Verification items for the finished model (mm, model axes). Face numbers are marked on the shaded views. A direction names the side the tool comes from. Coordinates: 2 decimals unless noted, no trailing zeros. Order: outer loops, then holes, each group sorted by start corner. A loop starts at its lowest first (then second) coordinate and runs counter-clockwise, first axis right, second up. Notation, with made-up numbers: M 10.25,57 L 56.25,57 A25 ccw 56.25,79 Z; hole C 69,65.25 d8. An arc over 180 degrees is marked long. Return JSON: item names as keys, results as strings.
Autodesk Inventor part; units mm, degrees
ref_plane "Work Plane1" through (30, 0, 0) normal (0, -0.5, 0.866) x (1, 0, 0)
ref_plane "YZ Plane" through (0, 0, 0) normal (1, 0, 0) x (0, 1, 0)
ref_plane "XZ Plane" through (0, 0, 0) normal (0, 1, 0) x (-1, 0, 0)
sketch "Skizze1" plane through (0, 0, 0) normal (0, 0, 1) x (1, 0, 0)
  line L0 (-0.19, 0) -> (25, 0)
  line L1 (25, 0) -> (25, 2.5)
  line L2 (25, 2.5) -> (1.6, 2.5)
  line L3 (1.6, 2.5) -> (1.1092, 2.5)
  line L4 (1.1092, 2.5) -> (0, 2.5)
  line L5 (0, 2.5) -> (0, 4.75)
  line L6 (0, 4.75) -> (-2.75, 4.75)
  line L7 (-2.75, 4.75) -> (-2.75, 1.7321)
  line L8 (-2.75, 1.7321) -> (-1.19, 1.7321)
  line L9 (-1.19, 1.7321) -> (-0.19, 0)
  line L10 (-8.3, 0) -> (30.55, 0)
  line L11 (0, -0.95) -> (0, 5.7)
  line L12 (1.6, 2.5) -> (0, 2.5) construction
  dimension "d0" = 23.4
  dimension "d1" = 0.4908
  dimension "d2" = 2.75
  dimension "d3" = 1.56
  dimension "d4" = 60
  dimension "d5" = 5
  dimension "d6" = 5
  dimension "d7" = 3.4641
  dimension "d8" = 9.5
  dimension "d19" = 25
revolve "Körper" add sketch "Skizze1" angle 360 about axis through (-0.19, 0, 0) along (1, 0, 0)
sketch "Skizze2" plane through (-2.75, 0, 0) normal (-1, 0, 0) x (0, 0, 1)
  circle A0 centre (0, 0) radius 1.7321
  line L0 (0, -6.65) -> (0, 6.65)
  line L1 (-6.65, 0) -> (6.65, 0)
  line L2 (1.7321, 0) -> (0.866, -1.5)
  line L3 (0.866, -1.5) -> (-0.866, -1.5)
  line L4 (-0.866, -1.5) -> (-1.7321, 0)
  line L5 (-1.7321, 0) -> (-0.866, 1.5)
  line L6 (-0.866, 1.5) -> (0.866, 1.5)
  line L7 (0.866, 1.5) -> (1.7321, 0)
extrude "Loch" add sketch "Skizze2" against normal up to next contours L7 A0 | A0 L2 | L6 L0 A0 | A0 L0 L3 | L0 L6 A0 | A0 L3 L0 | L4 A0 | A0 L5
fillet "Rundung1" radius 2.375 1 edges at (-2.75, -4.75, 0)
thread "Gewinde"
chamfer "Fase1" distance 0.4908 distance2 0.4908 1 edges at (25, -2.5, 0) measured on face at (25, 0.6587, -0.3326)
fillet "Rundung2" radius 0.2 1 edges at (0, -2.5, 0)
ref_plane "Work Plane1" through (30, 0, 0) normal (0, -0.5, 0.866) x (1, 0, 0)
sketch "Skizze4" plane through (25, 0, 0) normal (1, 0, 0) x (0, 0, -1)
  circle A0 centre (0, 0) radius 5
extrude "Extrusion3" cut sketch "Skizze4" against normal blind 3
chamfer "Fase3" distance 0.5 angle 45 1 edges at (22, -2.5, 0)
equation "\"d0\" = GEL"
equation "\"d1\" = GAL"
equation "\"d2\" = KOH"
equation "\"d3\" = INTI"
equation "\"d5\" = GD"
equation "\"d6\" = BDM"
equation "\"d7\" = 1.1547 * SW"
equation "\"d8\" = KOD"
equation "\"d19\" = NLG"
equation "\"d16\" = RR"
equation "\"d12\" = GEL"
equation "\"d14\" = -0.5 * SPD + 0.5 * GD"
equation "\"d15\" = GUL"
equation "\"d29\" = R"
equation "\"GD\" = NND"
equation "\"NLG\" = 25"
equation "\"GEL\" = 23.4"
equation "\"KOD\" = 9.5"
equation "\"KOH\" = 2.75"
equation "\"INTI\" = 1.56"
equation "\"GAL\" = 0.61345 * PTC"
equation "\"GUL\" = 0.61345 * PTC"
equation "\"BDM\" = NND"
equation "\"SW\" = 3"
equation "\"RR\" = 2.375"
equation "\"SPD\" = 4.01848"
equation "\"d28\" = R"
equation "\"R\" = 0.2"
equation "\"TOA\" = 30deg"
equation "\"THREADDIA\" = 5"
equation "\"KOD1\" = KOD - 2 * RR"
equation "\"PTC\" = 0.8"
equation "\"NND\" = 5"
equation "\"E0\" = 1.155 * SW"
equation "\"GD1\" = THREADDIA - 1.2269 * PTC"
properties part number "ANSI B18.3.4M - M5 x 0.8 x 25, BHSBHCSM" material "Stahl, weich"
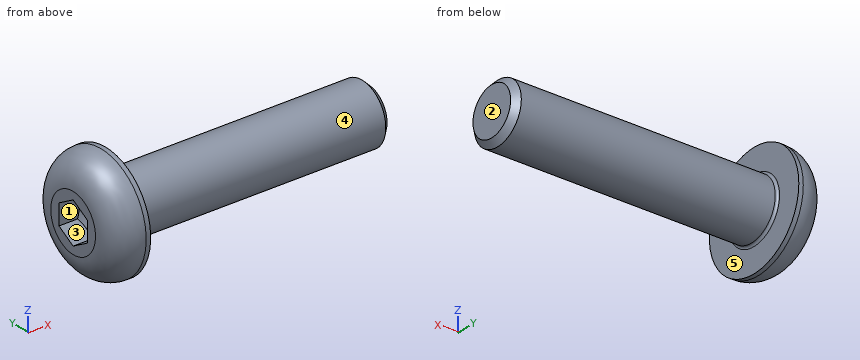
Q1. Draft check along Z on the marked faces 3, 4 and 5. Enter one of: pulls with the +Z half, pulls with the -Z half, needs draft (parallel to the pull), parting line crosses it, or undercut.
Values:
{"face 3": "undercut", "face 4": "parting line crosses it", "face 5": "needs draft"}
Q2. Cross-section at A-A, the plane x = 10.75. Record the boundary of the cut face in (y, z).
Values:
{"outline": "C 0,0 d5"}
Q3. Material ranges on line 1 along Z through (x, y) = (1, 2); line 2 along X through (y, z) = (0, -3.5); line 3 along Z through (x, y) = (3.75, -1), recorded low to high.
Values:
{"line 1": "-1.5 to 1.5", "line 2": "-2.47 to 0", "line 3": "-2.29 to 2.29"}
Q4. Tool access check on the marked faces 1 and 2. Record the directions out of +Z, -Z, +X, -X, +Y, -Y that give a thin tool (end or side, any length) a straight path to the whole face; none if there is none.
Values:
{"face 1": "-X", "face 2": "+Z, -Z, +X, +Y, -Y"}
Q5. Go/stop test with flat-tipped pins: pin 1 (1.9 mm diameter, centred on x = -1.5, z = 0.5, fed in from -Y); pin 2 (4 mm diameter, centred on x = 11, y = 2.5, fed in from +Z); pin 3 (2 mm diameter, centred on x = 17.5, z = 2.5, fed in from -Y). Record where each tip stops, or that it passes through.
Values:
{"pin 1": "y = -4.74", "pin 2": "z = 2.45", "pin 3": "y = -2"}
